Geometry: final body of the model. Coordinates: model frame, mm. A direction names the side the tool comes from. Give positions to 0.01 mm unless a question says otherwise; leave off trailing zeros. Write each loop counter-clockwise with the first axis right and the second up, starting at its lowest first coordinate (ties: lowest second). Pieces come first, ordered by that corner, then holes. Notation, with made-up numbers: M 8,-16 L 63,-16 A9 cw 63,-4 Z; hole C 32.5,74 d8. An arc over 180 degrees is marked long. Use a Markdown table: item, result. Add a question column.
(1) Pin query (flat end, axial travel): pin 1 Ø1.5 at (y, z) = (-7.5, 2.5) entering from -X; pin 2 Ø1 at (x, y) = (8.5, 0) entering from +Z; pin 3 Ø3.5 at (x, y) = (-1.5, -0.5) entering from -Z; pin 4 Ø4.5 at (x, y) = (-1.5, -9) entering from +Z. Return the tip coordinate at first contact, or that it passes through.
(2) Cut plane D-D (y = 0). Output: boundary loops of the cut face in (x, z), plus the area to 3 significant figures.
(3) Material intervals for L1, parallel to Y at x = -2, z = 1.7; L2, parallel to X at y = -11.5, z = 1.8; L3, parallel to Z at x = 3.25, y = -1, sorted ascending.
(4) Draft query along X for faces 5 (the flat face through (0, 0, 3.2)), 6 (the flat face through (-9.5, 1.5, 4.3)), 7 (the cylindrical face through (-1.608, -6.954, 1.387)). Return one class per face: released by +X, released by -X, zero draft, split by the parting line, or undercut.
(5) Cut plane A-A (y = -11.5). Output: boundary loops of the cut face in (x, z).
(6) Cut plane B-B (x = -2). Output: boundary loops of the cut face in (y, z), plus the area to 3 significant figures.
(7) Cut plane C-C (z = 1.95). Output: boundary loops of the cut face in (x, y).
(8) Reachability of faces 1 (the flat face through (0, -8, 2)), 2 (the flat face through (-2, -8, 2.3)), 3 (the flat face through (-1, -2.5, 2)), 4 (the flat face through (-4, -8, 2)) from +Z, -Z, +X, -X, +Y, -Y: full face, straight path, thin tool, end or side. Return the list, or none.
```python
from build123d import *

# Parameters (mm, degrees)
SKETCH_1_R          = 0.85
EXTRUDE_2_DEPTH     = 5.5
CUT_EXTRUDE_START   = 3.2
SKETCH_3_W          = 4
SKETCH_3_H          = 9.88
SKETCH_3_R          = 0.85
CUT_EXTRUDE_2_DEPTH = 3.2
CHAMFER_1_SIZE      = 1
CHAMFER_2_SIZE      = 1
CHAMFER_3_SIZE      = 0.5
SKETCH_4_R          = 0.85
CUT_EXTRUDE_3_DEPTH = 3.2
CHAMFER_4_SIZE      = 0.5
CHAMFER_4_SIZE2     = 0.566583589
CUT_EXTRUDE_4_DEPTH = 0.5


with BuildPart() as part:
    # 草图1 → 凸台-拉伸2 (new body)
    with BuildSketch(Plane.XY):
        Polygon((-10, 2), (10, 2), (10, -2), (0, -3.12), (0, -13), (-4, -13), (-4, -3.12), (-10, -2), align=None)
        with Locations((-7.5, 0)):
            Circle(SKETCH_1_R, mode=Mode.SUBTRACT)
        with Locations((8.5, 0)):
            Circle(SKETCH_1_R, mode=Mode.SUBTRACT)
        with Locations((-2, -11.5)):
            Circle(SKETCH_1_R, mode=Mode.SUBTRACT)
        with Locations((-2, -6.2)):
            Circle(SKETCH_1_R, mode=Mode.SUBTRACT)
    extrude(amount=EXTRUDE_2_DEPTH)

    # 草图3 → 切除-拉伸2 (cut)
    with BuildSketch(Plane(origin=(0, 0, 5.5), x_dir=(-1, 0, 0), z_dir=(0, 0, -1)).offset(CUT_EXTRUDE_START)):
        with Locations((2, -8.06)):
            Rectangle(SKETCH_3_W, SKETCH_3_H)
        with Locations((2, -11.5)):
            Circle(SKETCH_3_R, mode=Mode.SUBTRACT)
        with Locations((2, -6.2)):
            Circle(SKETCH_3_R, mode=Mode.SUBTRACT)
    extrude(amount=-CUT_EXTRUDE_2_DEPTH, mode=Mode.SUBTRACT)

    # 倒角1
    chamfer_1_edges = [part.edges().sort_by_distance(p)[0] for p in [
        (-2, -3.12, 2.3),
    ]]
    chamfer(chamfer_1_edges, length=CHAMFER_1_SIZE)

    # 倒角2
    chamfer_2_edges = [part.edges().sort_by_distance(p)[0] for p in [
        (-10, 2, 2.75),
        (10, 2, 2.75),
    ]]
    chamfer(chamfer_2_edges, length=CHAMFER_2_SIZE)

    # 倒角3
    chamfer_3_edges = [part.edges().sort_by_distance(p)[0] for p in [
        (0, -13, 1.15),
        (-4, -13, 1.15),
    ]]
    chamfer(chamfer_3_edges, length=CHAMFER_3_SIZE)

    # 草图4 → 切除-拉伸3 (cut)
    with BuildSketch(Plane.XY):
        Polygon((-10, -2.5), (10, -2.5), (10, 1), (9, 2), (-9, 2), (-10, 1), align=None)
        with Locations((8.5, 0)):
            Circle(SKETCH_4_R, mode=Mode.SUBTRACT)
        with Locations((-7.5, 0)):
            Circle(SKETCH_4_R, mode=Mode.SUBTRACT)
    extrude(amount=CUT_EXTRUDE_3_DEPTH, mode=Mode.SUBTRACT)

    # 倒角4
    chamfer_4_edges = [part.edges().sort_by_distance(p)[0] for p in [
        (10, -2, 4.35),
    ]]
    chamfer_4_side = [part.faces().sort_by_distance(p)[0] for p in [
        (4.028822055, -2.66877193, 3.153508772),
    ]]
    chamfer(chamfer_4_edges, length=CHAMFER_4_SIZE, length2=CHAMFER_4_SIZE2, reference=chamfer_4_side[0])

    # 草图5 → 切除-拉伸4 (cut)
    with BuildSketch(Plane(origin=(0, 0, 0), x_dir=(-1, 0, 0), z_dir=(0, 0, -1))):
        Polygon((4, -3.12), (7.321428571, -2.5), (-5.535714286, -2.5), (0, -3.12), (0, -12.5), (0.5, -13), (3.5, -13), (4, -12.5), align=None)
    extrude(amount=-CUT_EXTRUDE_4_DEPTH, mode=Mode.SUBTRACT)


solid = part.part
```
Answer list:
| question | item | result |
|---|---|---|
| 1 | pin 1 | x = -4 |
| 1 | pin 2 | through |
| 1 | pin 3 | z = 3.2 |
| 1 | pin 4 | z = 2.3 |
| 2 | outline | M -10,3.2 L -8.35,3.2 L -8.35,5.5 L -10,5.5 Z; M -6.65,3.2 L 7.65,3.2 L 7.65,5.5 L -6.65,5.5 Z; M 9.35,3.2 L 10,3.2 L 10,5.5 L 9.35,5.5 Z |
| 2 | area | 38.2 mm² |
| 3 | L1 | -13 to -12.35, -10.65 to -7.05, -5.35 to -2.5 |
| 3 | L2 | -4 to -2.85, -1.15 to 0 |
| 3 | L3 | 3.2 to 5.5 |
| 4 | face 5 | zero draft |
| 4 | face 6 | released by -X |
| 4 | face 7 | undercut |
| 5 | outline | M -4,0.5 L -2.85,0.5 L -2.85,2.3 L -4,2.3 Z; M -1.15,0.5 L 0,0.5 L 0,2.3 L -1.15,2.3 Z |
| 6 | outline | M -13,0.5 L -12.35,0.5 L -12.35,2.3 L -13,2.3 Z; M -10.65,0.5 L -7.05,0.5 L -7.05,2.3 L -10.65,2.3 Z; M -5.35,0.5 L -2.5,0.5 L -2.5,3.2 L 2,3.2 L 2,5.5 L -3.12,5.5 L -3.12,3.3 L -4.12,2.3 L -5.35,2.3 Z |
| 6 | area | 25.6 mm² |
| 7 | outline | M -7.32,-2.5 L -4,-3.12 L -4,-12.5 L -3.5,-13 L -0.5,-13 L 0,-12.5 L 0,-3.12 L 5.54,-2.5 Z; hole C -2,-11.5 d1.7; hole C -2,-6.2 d1.7 |
| 8 | face 1 | +Z, -Z, +X, -Y |
| 8 | face 2 | +Z, +X, -X, -Y |
| 8 | face 3 | -Z, +X, -X, +Y |
| 8 | face 4 | +Z, -Z, -X, -Y |
